CAD build for the part. Positions are in the model's coordinates, mm. A direction names the side the tool comes from. Give positions to 0.01 mm unless a question says otherwise; leave off trailing zeros. Loops run counter-clockwise (first coordinate to the right, second up) from the corner with the lowest first, then second, coordinate; pieces in that order, holes last. Notation, with made-up numbers: M 76,-17 L 104,-17 A23 ccw 104,12 Z; hole C 66,60 d3. An arc over 180 degrees is marked long. Answer as CSV lines item,"result".
from build123d import *

# Parameters (mm, degrees)
F0_R     = 7.5
F1_DEPTH = 10
F3_DEPTH = 2.5
F4_R     = 2


with BuildPart() as f1:
    # F0 (on Top) → F1 (new body)
    with BuildSketch(Plane.XY):
        Circle(F0_R)
    extrude(amount=F1_DEPTH)

    # F2 (on Front) → F3 (join, symmetric)
    with BuildSketch(Plane.XZ):
        Polygon((2.5, 22), (-2.5, 22), (-2.5, 18), (-7.5, 18), (-7.5, 14), (-2.5, 14), (-2.5, 10), (2.5, 10), (2.5, 14), (7.5, 14), (7.5, 18), (2.5, 18), align=None)
    extrude(amount=F3_DEPTH, both=True)

    # F4
    f4_edges = [f1.edges().sort_by_distance(p)[0] for p in [
        (-7.5, 0, 10),
    ]]
    fillet(f4_edges, radius=F4_R)


solid = f1.part
1) Band-saw the part on B-B on x = 0. Give the cut face in (y, z).
Answer below:
outline,"M -7.5,0 L 7.5,0 L 7.5,8 A2 ccw 5.5,10 L 2.5,10 L 2.5,22 L -2.5,22 L -2.5,10 L -5.5,10 A2 ccw -7.5,8 Z"
2) Band-saw the part on D-D on z = 12.25. Give the cut face in (x, y).
Answer below:
outline,"M -2.5,-2.5 L 2.5,-2.5 L 2.5,2.5 L -2.5,2.5 Z"
3) Flat gauge pins, fed straight in: pin 1 (6 mm diameter, centred on x = 1.5, z = 15.5, fed in from +Y); pin 2 (1.5 mm diameter, centred on x = -6, y = 0, fed in from +Z); pin 3 (1.2 mm diameter, centred on y = 0, z = 21, fed in from -X). Where does each tip first touch, or does it go through?
Answer below:
pin 1,"stops at y = 2.5"
pin 2,"stops at z = 18"
pin 3,"stops at x = -2.5"
4) Drill centre lines: line 1 (Z direction, x = 4.25, y = -2); line 2 (Z direction, x = 1, y = 3.5); line 3 (Z direction, x = 5.75, y = 2). Where is each one in solid material? Low to high. Write a range as from..to.
Answer below:
line 1,"z = 0..10, 14..18"
line 2,"z = 0..10"
line 3,"z = 0..9.91, 14..18"
5) Band-saw the part on A-A on y = 0. Give the cut face in (x, z), and give its area (3 significant figures).
Answer below:
outline,"M -7.5,0 L 7.5,0 L 7.5,8 A2 ccw 5.5,10 L 2.5,10 L 2.5,14 L 7.5,14 L 7.5,18 L 2.5,18 L 2.5,22 L -2.5,22 L -2.5,18 L -7.5,18 L -7.5,14 L -2.5,14 L -2.5,10 L -5.5,10 A2 ccw -7.5,8 Z"
area,"248 mm^2"
6) Which spindle directions (+Z, -Z, +X, -X, +Y, -Y) get a long thin tool onto all of the face, cutting with end or side? Do faces 1 (the face through (0, 2.5, 16)), 2 (the face through (-5, 0, 14)), 3 (the face through (0, -2.5, 16)), 4 (the face through (2.5, 0, 12)). Say none if no direction does.
Answer below:
face 1,"+Z, +X, -X, +Y"
face 2,"-X, +Y, -Y"
face 3,"+Z, +X, -X, -Y"
face 4,"+X, +Y, -Y"
7) Mould opens along Z. For faces 5 (the face through (-3, 0, 10)), 6 (the face through (5, 0, 18)), 7 (the face through (0, 0, 0)) say: +Z half, -Z half, draft (parallel to the pull), parting line (faces both ways), or undercut.
Answer below:
face 5,"undercut"
face 6,"+Z half"
face 7,"-Z half"
8) Band-saw the part on C-C on z = 15.5. Give the cut face in (x, y), and give its area (3 significant figures).
Answer below:
outline,"M -7.5,-2.5 L 7.5,-2.5 L 7.5,2.5 L -7.5,2.5 Z"
area,"75.0 mm^2"
